Input: part model. Units: mm. Frame: model coordinates. Round coordinates to 2 decimals unless told otherwise and drop trailing zeros. Order: outer loops, then holes, each group sorted by start corner. A loop starts at its lowest first (then second) coordinate and runs counter-clockwise, first axis right, second up. Notation, with made-up numbers: (50, 21.25) - (88, 21.25) arc R22 ccw to (88, 34.25) - close; hole circle Ø1 at (6.25, 63). An arc over 180 degrees is marked (long way). One line per item, written item: value. Start each with the question number.
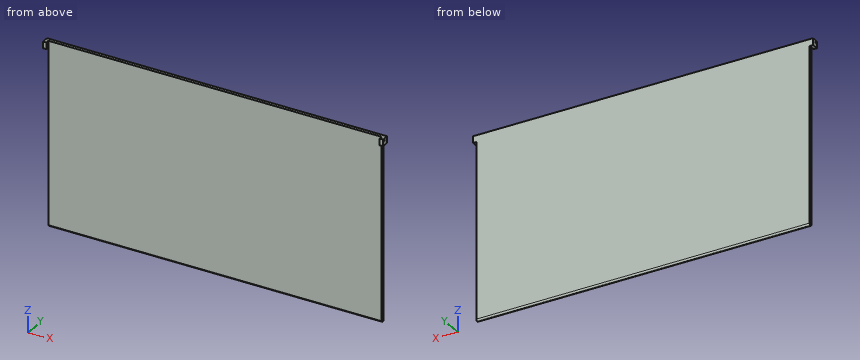
from build123d import *

# Parameters (mm, degrees)
SKETCH1_W           = 200
SKETCH1_H           = 110
BOSS_EXTRUDE1_DEPTH = 2
FILLET1_R           = 1
SKETCH3_W           = 4
SKETCH3_H           = 4
SKETCH3_R           = 0.5
BOSS_EXTRUDE2_DEPTH = 2
BOSS_EXTRUDE3_START = 2
SKETCH4_W           = 4
SKETCH4_H           = 4
SKETCH4_R           = 0.5
BOSS_EXTRUDE3_DEPTH = 2


with BuildPart() as part:
    # Sketch1 → Boss-Extrude1 (new body)
    with BuildSketch(Plane(origin=(0, 0, 0), x_dir=(1, 0, 0), z_dir=(0, 1, 0))):
        Rectangle(SKETCH1_W, SKETCH1_H)
    extrude(amount=BOSS_EXTRUDE1_DEPTH)

    # Fillet1
    fillet1_edges = [part.edges().sort_by_distance(p)[0] for p in [
        (0, 0, -55),
        (0, 2, -55),
    ]]
    fillet(fillet1_edges, radius=FILLET1_R - 0.0001)  # a hair under: the kernel refuses the full size

    # Sketch3 → Boss-Extrude2 (add)
    with BuildSketch(Plane.ZY.offset(100)):
        with Locations((53, 0)):
            Rectangle(SKETCH3_W, SKETCH3_H)
        with Locations((54, -1.003505598)):
            Circle(SKETCH3_R, mode=Mode.SUBTRACT)
    extrude(amount=BOSS_EXTRUDE2_DEPTH)

    # Sketch4 → Boss-Extrude3 (add)
    with BuildSketch(Plane(origin=(100, 0, 0), x_dir=(0, 0, -1), z_dir=(1, 0, 0)).offset(BOSS_EXTRUDE3_START)):
        with Locations((-53, 0)):
            Rectangle(SKETCH4_W, SKETCH4_H)
        with Locations(Location((-54, -1.003505598, 0), (0, 0, 180))):
            Circle(SKETCH4_R, mode=Mode.SUBTRACT)
    extrude(amount=-BOSS_EXTRUDE3_DEPTH)


solid = part.part
Item 1: First-contact query: pin 1 Ø2 at (x, y) = (31.5, -0.5) entering from -Z; pin 2 Ø0.6 at (y, z) = (1.5, -25.5) entering from -X; pin 3 Ø1 at (x, z) = (-2.5, -8.5) entering from -Y. Flat tips, straight axial feed; report the tip coordinate or a pass-through.
Item 2: Section query B-B on z = -46. Return loops of the section in (x, y), and give its area (3 significant figures).
Item 3: Line query: L1, parallel to Z at x = 6.5, y = 1.3; L2, parallel to Y at x = -101.45, z = 54; L3, parallel to Y at x = -18.5, z = -2.5. Output: solid intervals per line, ascending.
Geometry results:
1. pin 1: stops at z = -54.87
1. pin 2: stops at x = -100
1. pin 3: stops at y = 0
2. outline: (-100, 0) - (100, 0) - (100, 2) - (-100, 2) - close
2. area: 400 mm^2
3. L1: z = -54.95 to 55
3. L2: y = -2 to -1.5, -0.5 to 2
3. L3: y = 0 to 2
